Read the model definition and answer for the solid it produces. Units are mm, in the model's axes. A direction names the side the tool comes from. Round coordinates to 2 decimals unless told otherwise and drop trailing zeros. Loops run counter-clockwise (first coordinate to the right, second up) from the corner with the lowest first, then second, coordinate; pieces in that order, holes last. Notation, with made-up numbers: (88.25, 10.5) -> (104.25, 10.5) arc R13 ccw to (104.25, 27.5) -> close; hole circle Ø10 at (41.25, 24.5). An arc over 180 degrees is marked (long way). Put each result on its own line as item: value.
from build123d import *

# Parameters (mm, degrees)
ESBO_O1_R                = 43.5
RESSALTO_EXTRUS_O1_DEPTH = 5
ESBO_O2_R                = 38.5
RESSALTO_EXTRUS_O2_DEPTH = 15
ESBO_O3_R                = 35.5
CORTE_EXTRUS_O1_DEPTH    = 21
CORTE_EXTRUS_O2_DEPTH    = 21


with BuildPart() as part:
    # Esboço1 → Ressalto-extrusão1 (new body)
    with BuildSketch(Plane.XY):
        Circle(ESBO_O1_R)
    extrude(amount=RESSALTO_EXTRUS_O1_DEPTH)

    # Esboço2 → Ressalto-extrusão2 (add)
    with BuildSketch(Plane.XY.offset(5)):
        Circle(ESBO_O2_R)
    extrude(amount=RESSALTO_EXTRUS_O2_DEPTH)

    # Esboço3 → Corte-extrusão1 (cut, through all)
    with BuildSketch(Plane.XY.offset(20)):
        Circle(ESBO_O3_R)
    extrude(amount=-CORTE_EXTRUS_O1_DEPTH, mode=Mode.SUBTRACT)

    # Esboço4 → Corte-extrusão2 (cut, through all)
    with BuildSketch(Plane(origin=(0, 0, 0), x_dir=(-1, 0, 0), z_dir=(0, 0, -1))):
        with BuildLine():
            Line((0, 0), (24.950574981, 35.633113927))
            ThreePointArc((24.950574981, 35.633113927), (0, 43.5), (-24.950574981, 35.633113927))
            Line((-24.950574981, 35.633113927), (0, 0))
        make_face()
    extrude(amount=-CORTE_EXTRUS_O2_DEPTH, mode=Mode.SUBTRACT)


solid = part.part
Item 1: The part is cut by section C-C (x = 0). Determine the outline of the cut face in (y, z), then the cut area to 3 significant figures.
Derived:
outline: (-43.5, 0) -> (-35.5, 0) -> (-35.5, 20) -> (-38.5, 20) -> (-38.5, 5) -> (-43.5, 5) -> close
area: 85.0 mm^2
Item 2: For a pull along X with two mould halves and no side action, classify faces 3 (the flat face through (-12, -34, 20)), 4 (the cylindrical face through (-1.541, -43.473, 2.465)), 5 (the flat face through (21.67, 30.95, 7.64)), 6 (the flat face through (-21.6, 30.85, 7.64)) as pulls with the +X half, pulls with the -X half, needs draft (parallel to the pull), parting line crosses it, or undercut.
Derived:
face 3: needs draft
face 4: parting line crosses it
face 5: undercut
face 6: undercut
Item 3: The part is cut by section D-D (z = 9.75). Determine the outline of the cut face in (x, y).
Derived:
outline: (-22.08, 31.54) arc R38.5 ccw (long way) to (22.08, 31.54) -> (20.36, 29.08) arc R35.5 cw (long way) to (-20.36, 29.08) -> close
Item 4: Find the intervals of material crossed by line 1 along X through (y, z) = (0, 13.25); line 2 along X through (y, z) = (21.5, 6); line 3 along Y through (x, z) = (0, 8), in increasing order.
Derived:
line 1: x = -38.5 to -35.5, 35.5 to 38.5
line 2: x = -31.94 to -28.25, 28.25 to 31.94
line 3: y = -38.5 to -35.5
Item 5: Which of the six approach directions +Z, -Z, +X, -X, +Y, -Y give full straight-line access (tool end or side, diameter ignored) to faces 1 (the cylindrical face through (-1.258, -35.478, 10.14)), 2 (the flat face through (0, -39, 5))?
Derived:
face 1: +Z, -Z
face 2: +Z
Item 6: The part is cut by section A-A (y = 2). Determine the outline of the cut face in (x, z), then the cut area to 3 significant figures.
Derived:
outline: (-43.45, 0) -> (-35.44, 0) -> (-35.44, 20) -> (-38.45, 20) -> (-38.45, 5) -> (-43.45, 5) -> close; (35.44, 0) -> (43.45, 0) -> (43.45, 5) -> (38.45, 5) -> (38.45, 20) -> (35.44, 20) -> close
area: 170 mm^2
Item 7: Flat-ended cylindrical pins translate along their axes: pin 1 Ø10 at (x, z) = (7, 11) entering from -Y; pin 2 Ø4 at (y, z) = (5.5, 14) entering from +X; pin 3 Ø8 at (x, z) = (-24, 13.5) entering from +Y. Find the tip coordinate at first contact, or state that the pin passes through.
Derived:
pin 1: stops at y = -38.45
pin 2: stops at x = 38.34
pin 3: stops at y = 31.54
Item 8: The part is cut by section B-B (x = 28.5). Determine the outline of the cut face in (y, z).
Derived:
outline: (-32.86, 0) -> (-21.17, 0) -> (-21.17, 20) -> (-25.88, 20) -> (-25.88, 5) -> (-32.86, 5) -> close; (21.17, 0) -> (32.86, 0) -> (32.86, 5) -> (25.88, 5) -> (25.88, 20) -> (21.17, 20) -> close
